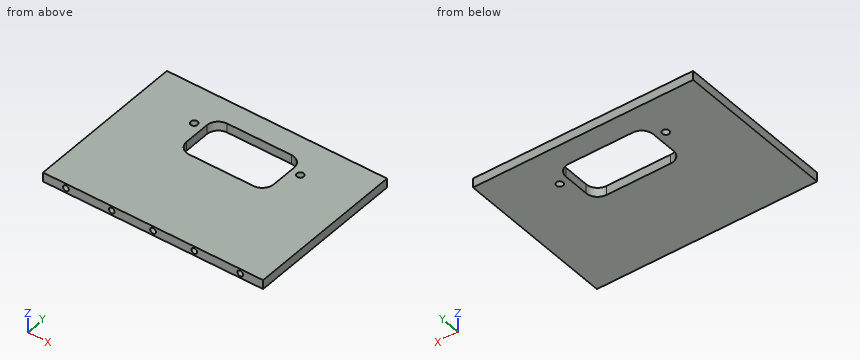
```python
from build123d import *

# Parameters (mm, degrees)
ESBO_O1_W                = 96.01
ESBO_O1_H                = 70
RESSALTO_EXTRUS_O1_DEPTH = 4
ESBO_O2_R                = 1.25
CORTE_EXTRUS_O1_DEPTH    = 12
ESBO_O3_R                = 1.5
ESBO_O3_W                = 38.01
ESBO_O3_H                = 21.381971147
CORTE_EXTRUS_O2_DEPTH    = 10
FILETE1_R                = 5


with BuildPart() as part:
    # Esboço1 → Ressalto-extrusão1 (new body)
    with BuildSketch(Plane.XY):
        with Locations((48.005, -35)):
            Rectangle(ESBO_O1_W, ESBO_O1_H)
    extrude(amount=RESSALTO_EXTRUS_O1_DEPTH)

    # Esboço2 → Corte-extrusão1 (cut)
    with BuildSketch(Plane(origin=(0, -70, 0), x_dir=(-1, 0, 0), z_dir=(0, -1, 0))):
        with Locations((-48.005, -2)):
            Circle(ESBO_O2_R)
        with Locations((-10, -2)):
            Circle(ESBO_O2_R)
        with Locations((-30, -2)):
            Circle(ESBO_O2_R)
        with Locations((-66.01, -2)):
            Circle(ESBO_O2_R)
        with Locations((-86.01, -2)):
            Circle(ESBO_O2_R)
    extrude(amount=-CORTE_EXTRUS_O1_DEPTH, mode=Mode.SUBTRACT)

    # Esboço3 → Corte-extrusão2 (cut)
    with BuildSketch(Plane.XY.offset(4)):
        with Locations((24.85, -16.78)):
            Circle(ESBO_O3_R)
        with Locations((71.16, -16.78)):
            Circle(ESBO_O3_R)
        with Locations((48.005, -20.690985574)):
            Rectangle(ESBO_O3_W, ESBO_O3_H)
    extrude(amount=-CORTE_EXTRUS_O2_DEPTH, mode=Mode.SUBTRACT)

    # Filete1
    filete1_edges = [part.edges().sort_by_distance(p)[0] for p in [
        (29, -31.381971147, 2),
        (29, -10, 2),
        (67.01, -10, 2),
        (67.01, -31.381971147, 2),
    ]]
    fillet(filete1_edges, radius=FILETE1_R)


solid = part.part
```
Part model, mm, in its own coordinate system. Round coordinates to 2 decimals unless told otherwise and drop trailing zeros. Write each loop counter-clockwise with the first axis right and the second up, starting at its lowest first coordinate (ties: lowest second). Pieces come first, ordered by that corner, then holes. Notation, with made-up numbers: M 40,12 L 84,12 A30 ccw 84,34 Z; hole C -26.75,-18 d1. An arc over 180 degrees is marked long. One line per question, with ' | ' between items.
(1) Saw through at B-B on x = 86.01. Write the cut outline in (y, z), then the cut area to 3 significant figures.
Answer key:
outline: M -70,0 L 0,0 L 0,4 L -70,4 L -70,3.25 L -58,3.25 L -58,0.75 L -70,0.75 Z | area: 250 mm^2
(2) Saw through at C-C on y = -29. Write the cut outline in (x, z).
Answer key:
outline: M 0,0 L 29.74,0 L 29.74,4 L 0,4 Z; M 66.27,0 L 96.01,0 L 96.01,4 L 66.27,4 Z
(3) Saw through at A-A on x = 71.16. Write the cut outline in (y, z), then the cut area to 3 significant figures.
Answer key:
outline: M -70,0 L -18.28,0 L -18.28,4 L -70,4 Z; M -15.28,0 L 0,0 L 0,4 L -15.28,4 Z | area: 268 mm^2
(4) Pin check, flat tip, straight feed: pin 1 (2 mm diameter, centred on x = 10, z = 2, fed in from -Y). Stop position of the tip, or through.
Answer key:
pin 1: stops at y = -58
(5) Saw through at D-D on x = 30. Write the cut outline in (y, z), then the cut area to 3 significant figures.
Answer key:
outline: M -70,0 L -29.38,0 L -29.38,4 L -70,4 L -70,3.25 L -58,3.25 L -58,0.75 L -70,0.75 Z; M -12,0 L 0,0 L 0,4 L -12,4 Z | area: 180 mm^2
(6) Probe line 1 along X through (y, z) = (-64, 2) (3 decimals); line 2 along X through (y, z) = (-20, 3.8); line 3 along Y through (x, z) = (58.5, 2.8). List the from-to ranges inside material, lowest first.
Answer key:
line 1: x = 0 to 8.75, 11.25 to 28.75, 31.25 to 46.755, 49.255 to 64.76, 67.26 to 84.76, 87.26 to 96.01 | line 2: x = 0 to 29, 67.01 to 96.01 | line 3: y = -70 to -31.38, -10 to 0
